from build123d import *

# Parameters (mm, degrees)
ESQUISSE1_R                  = 11
BOSS_EXTRU_1_DEPTH           = 5
ESQUISSE3_R                  = 14
BOSS_EXTRU_3_DEPTH           = 8.35
ENL_V_MAT_EXTRU_1_DEPTH      = 24.879332068
ENL_V_MAT_EXTRU_1_DEPTH_BACK = 24.879332068
ESQUISSE5_R                  = 1.25
BOSS_EXTRU_6_DEPTH           = 2
R_P_TITION_CIRCULAIRE1_COUNT = 3
BOSS_EXTRU_8_DEPTH           = 4.5
R_P_TITION_CIRCULAIRE3_COUNT = 3
D_GAGEMENT_M51_D             = 5.5
D_GAGEMENT_M51_CSINK_D       = 5.55
D_GAGEMENT_M51_CSINK_ANGLE   = 90
R_P_TITION_CIRCULAIRE4_COUNT = 3


with BuildPart() as part:
    # Esquisse1 → Boss.-Extru.1 (new body)
    with BuildSketch(Plane(origin=(0, 0, 0), x_dir=(1, 0, 0), z_dir=(0, 1, 0))):
        with Locations(Location((0, 0, 0), (0, 0, 270))):
            Circle(ESQUISSE1_R)
    extrude(amount=BOSS_EXTRU_1_DEPTH)

    # Esquisse3 → Boss.-Extru.3 (add)
    with BuildSketch(Plane.XZ):
        with Locations(Location((0, 0, 0), (0, 0, 270))):
            Circle(ESQUISSE3_R)
    extrude(amount=BOSS_EXTRU_3_DEPTH)

    # Esquisse5 → Enlèv. mat.-Extru.1 (cut, two sides: drawn at the far end of the back side and taken through both)
    with BuildSketch(Plane.XZ.offset(8.35).offset(-ENL_V_MAT_EXTRU_1_DEPTH_BACK)):
        with Locations(Location((0, 0, 0), (0, 0, 270))):
            Circle(ESQUISSE5_R)
    extrude(amount=ENL_V_MAT_EXTRU_1_DEPTH + ENL_V_MAT_EXTRU_1_DEPTH_BACK, mode=Mode.SUBTRACT)

    # Esquisse8 → Boss.-Extru.6 (add)
    with BuildSketch(Plane.XZ.offset(8.35)):
        with BuildLine():
            Line((-4.9, 28.05), (4.9, 28.05))
            Line((4.9, 28.05), (4.9, 5.678027827))
            ThreePointArc((4.9, 5.678027827), (0, 7.5), (-4.9, 5.678027827))
            Line((-4.9, 5.678027827), (-4.9, 28.05))
        make_face()
    boss_extru_6 = extrude(amount=-BOSS_EXTRU_6_DEPTH)

    # Répétition circulaire1: Boss.-Extru.6 ×3 about axis
    r_p_tition_circulaire1_axis = Axis((0, 0, 0), (0, 1, 0))
    for i in range(1, R_P_TITION_CIRCULAIRE1_COUNT):
        add(boss_extru_6.rotate(r_p_tition_circulaire1_axis, i * 360 / R_P_TITION_CIRCULAIRE1_COUNT))

    # Esquisse13 → Boss.-Extru.8 (add)
    with BuildSketch(Plane(origin=(0, -6.35, 0), x_dir=(1, 0, 0), z_dir=(0, 1, 0))):
        Polygon((-23.067012576, 16.146762239), (-25.517012576, 11.903237761), (-23.067012576, 7.659713282), (-18.167012576, 7.659713282), (-15.717012576, 11.903237761), (-18.167012576, 16.146762239), align=None)
    boss_extru_8 = extrude(amount=BOSS_EXTRU_8_DEPTH)

    # Répétition circulaire3: Boss.-Extru.8 ×3 about axis
    r_p_tition_circulaire3_axis = Axis((0, 0, 0), (0, 1, 0))
    for i in range(1, R_P_TITION_CIRCULAIRE3_COUNT):
        add(boss_extru_8.rotate(r_p_tition_circulaire3_axis, i * 360 / R_P_TITION_CIRCULAIRE3_COUNT))

    # Dégagement M51 (through all)
    with Locations(Plane(origin=(-20.617012576, -1.85, -11.903237761), x_dir=(0, 0, 1), z_dir=(0, 1, 0))):
        with Locations((0, 0)):
            d_gagement_m51 = CounterSinkHole(D_GAGEMENT_M51_D / 2, D_GAGEMENT_M51_CSINK_D / 2, counter_sink_angle=D_GAGEMENT_M51_CSINK_ANGLE)

    # Répétition circulaire4: Dégagement M51 ×3 about axis
    r_p_tition_circulaire4_axis = Axis((0, 0, 0), (0, 1, 0))
    for i in range(1, R_P_TITION_CIRCULAIRE4_COUNT):
        add(d_gagement_m51.rotate(r_p_tition_circulaire4_axis, i * 360 / R_P_TITION_CIRCULAIRE4_COUNT), mode=Mode.SUBTRACT)


solid = part.part
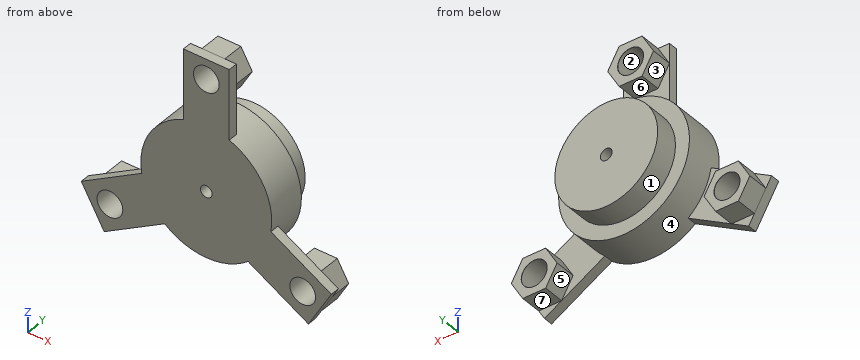
The model under review builds one solid part; all positions refer to its coordinate system, in mm. Face numbers are marked on the shaded views. A direction names the side the tool comes from. Give positions to 0.01 mm unless a question says otherwise; leave off trailing zeros. Write each loop counter-clockwise with the first axis right and the second up, starting at its lowest first coordinate (ties: lowest second). Pieces come first, ordered by that corner, then holes. Notation, with made-up numbers: M 73.5,61.25 L 106.5,61.25 A24 cw 106.5,97.25 Z; hole C -19,-18 d11. An arc over 180 degrees is marked long. One line per question, with ' | ' between items. Start each with the question number.
Item 1: We need section C-C on y = -5.25. Write out the cut boundary in (x, z), plus the area to 3 significant figures.
Item 2: We need section A-A on x = 0. Write out the cut boundary in (y, z) (3 decimals), plus the area to 3 significant figures.
Item 3: For the marked faces 4, 5, 6 and 7, list the 3-axis set-ups (+Z, -Z, +X, -X, +Y, -Y) from which the entire face can be reached by the end or side of a thin tool; tool diameter is ignored.
Item 4: Draft analysis for pull direction X (two halves, no side actions). For the marked faces 1, 2 and 3, state which applies: released by +X, released by -X, zero draft, split by the parting line, or undercut.
Item 5: Wall thickness on line 1 (Z direction, x = 0, y = -2); line 2 (Z direction, x = 0, y = -6.5); line 3 (X direction, y = -0.75, z = 0): over which ranges is each line inside the solid? List them lowest first. Write a range as from..to.
Item 6: For pin 1 (1.5 mm diameter, centred on y = 2.5, z = -8, fed in from -X); pin 2 (9.5 mm diameter, centred on x = 0, z = 25.5, fed in from +Y); pin 3 (1.3 mm diameter, centred on x = 19.5, y = -3, fed in from -Z); pin 4 (9 mm diameter, centred on x = 20.62, z = -11.9, fed in from -Y), all flat-tipped, find the tip position at first contact; note any pin that passes through.
Item 7: We need section D-D on y = 1. Write out the cut boundary in (x, z), plus the area to 3 significant figures.
Item 8: We need section B-B on z = 0. Write out the cut boundary in (x, y), plus the area to 3 significant figures.
Results found:
1) outline: M -25.52,-11.9 L -23.07,-16.15 L -18.17,-16.15 L -15.72,-11.9 L -18.17,-7.66 L -23.07,-7.66 Z; C 0,0 d28; M -4.9,23.81 L -2.45,19.56 L 2.45,19.56 L 4.9,23.81 L 2.45,28.05 L -2.45,28.05 Z; M 15.72,-11.9 L 18.17,-16.15 L 23.07,-16.15 L 25.52,-11.9 L 23.07,-7.66 L 18.17,-7.66 Z; hole C -20.62,-11.9 d5.5; hole C 0,23.81 d5.5; hole C 0,0 d2.5; hole C 20.62,-11.9 d5.5 | area: 727 mm2
2) outline: M -8.35,-14 L 0,-14 L 0,-11 L 5,-11 L 5,-1.25 L -8.35,-1.25 Z; M -8.35,1.25 L 5,1.25 L 5,11 L 0,11 L 0,14 L -6.35,14 L -6.35,19.563 L -1.85,19.563 L -1.85,21.031 L -1.875,21.056 L -8.35,21.056 Z; M -8.35,26.556 L -1.875,26.556 L -1.85,26.581 L -1.85,28.05 L -8.35,28.05 Z | area: 341 mm2
3) face 4: +Y | face 5: -Z, +Y | face 6: +X, -X, +Y | face 7: -Z, +X, -X, +Y
4) face 1: split by the parting line | face 2: undercut | face 3: released by -X
5) line 1: z = -14..-1.25, 1.25..14, 19.56..21.06, 26.56..28.05 | line 2: z = -14..-1.25, 1.25..21.06, 26.56..28.05 | line 3: x = -14..-1.25, 1.25..14
6) pin 1: stops at x = -8.27 | pin 2: stops at y = -1.85 | pin 3: stops at z = -16.15 | pin 4: stops at y = -8.35
7) outline: C 0,0 d22; hole C 0,0 d2.5 | area: 375 mm2
8) outline: M -14,-8.35 L -1.25,-8.35 L -1.25,5 L -11,5 L -11,0 L -14,0 Z; M 1.25,-8.35 L 14,-8.35 L 14,0 L 11,0 L 11,5 L 1.25,5 Z | area: 310 mm2
